The figure shows three views and two pictorial views of one solid part (mm, origin at its lowest corner). Answer the questions. A direction names the side the tool comes from. Round coordinates to 2 decimals unless told otherwise and drop trailing zeros. Write each loop counter-clockwise with the first axis right and the second up, starting at its lowest first coordinate (ties: lowest second). Pieces come first, ordered by that corner, then holes. Notation, with made-up numbers: M 57.5,83.25 L 99.5,83.25 A34 cw 99.5,119.25 Z; hole C -15.75,-14.75 d6. An arc over 180 degrees is marked long. Answer in a Markdown table with one row per item.
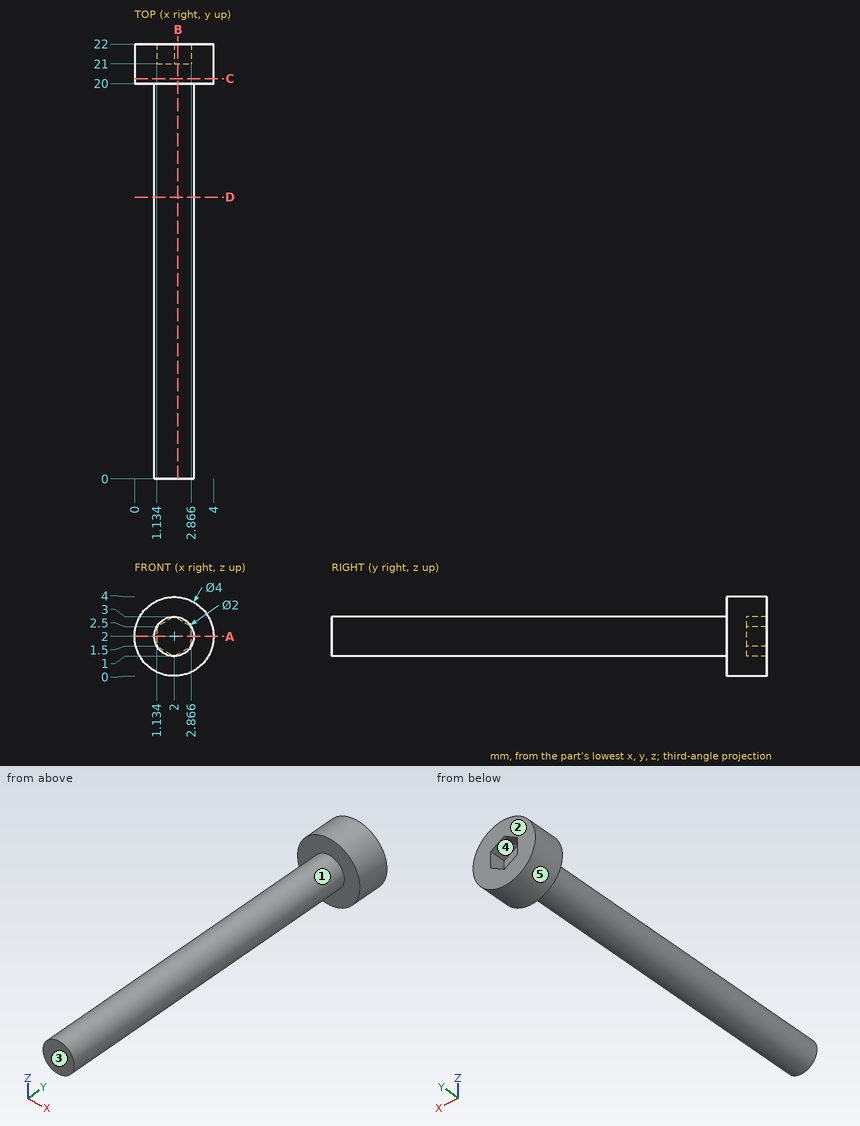
1. The part is cut by section A-A (z = 2). Determine the outline of the cut face in (x, y), plus the area to 3 significant figures.
Calculated:
| item | result |
|---|---|
| outline | M 0,20 L 1,20 L 1,0 L 3,0 L 3,20 L 4,20 L 4,22 L 2.87,22 L 2.87,21 L 1.13,21 L 1.13,22 L 0,22 Z |
| area | 46.3 mm² |
2. The part is cut by section C-C (y = 20.25). Determine the outline of the cut face in (x, z), plus the area to 3 significant figures.
Calculated:
| item | result |
|---|---|
| outline | C 2,2 d4 |
| area | 12.6 mm² |
3. Given pin 1 (1.5 mm diameter, centred on y = 3.5, z = 1, fed in from -X); pin 2 (1.5 mm diameter, centred on x = 2.5, y = 11, fed in from -Z), each flat-ended and moving along its own axis, determine where each tip first touches the part or whether it passes through.
Calculated:
| item | result |
|---|---|
| pin 1 | stops at x = 1.03 |
| pin 2 | stops at z = 1 |
4. The part is cut by section B-B (x = 2.2). Determine the outline of the cut face in (y, z), plus the area to 3 significant figures.
Calculated:
| item | result |
|---|---|
| outline | M 0,1.02 L 20,1.02 L 20,0.01 L 22,0.01 L 22,1.12 L 21,1.12 L 21,2.88 L 22,2.88 L 22,3.99 L 20,3.99 L 20,2.98 L 0,2.98 Z |
| area | 45.4 mm² |
5. A tool of negligible diameter and unlimited length cuts with its end or side. For the marked faces 1 and 2, from which of +Z, -Z, +X, -X, +Y, -Y can it reach the whole face along a straight path? Write none if from no direction.
Calculated:
| item | result |
|---|---|
| face 1 | -Y |
| face 2 | +Z, -Z, +X, -X, +Y |
6. Consider line 1 along Y through (x, z) = (1.6, 0.55); line 2 along Y through (x, z) = (1.75, 1.6); line 3 along Z through (x, y) = (1.15, 15). Determine where each line is inside the solid, lowest interval first. Write a range as from..to.
Calculated:
| item | result |
|---|---|
| line 1 | y = 20..22 |
| line 2 | y = 0..21 |
| line 3 | z = 1.47..2.53 |
7. Determine the mould class of the marked faces 3, 4 and 5 for opening direction X: released by +X, released by -X, zero draft, split by the parting line, or undercut.
Calculated:
| item | result |
|---|---|
| face 3 | zero draft |
| face 4 | undercut |
| face 5 | split by the parting line |
8. The part is cut by section D-D (y = 14.25). Determine the outline of the cut face in (x, z), plus the area to 3 significant figures.
Calculated:
| item | result |
|---|---|
| outline | C 2,2 d2 |
| area | 3.14 mm² |
